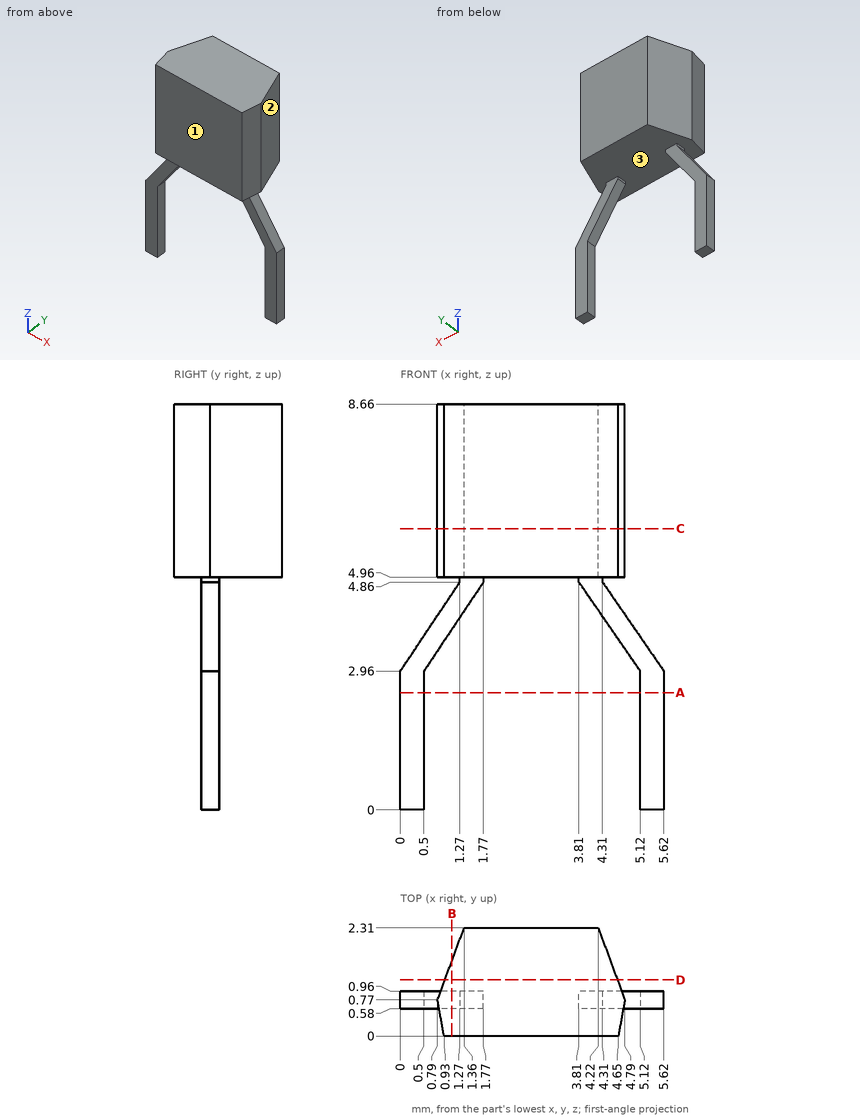
Part print with two shaded views. Sizes in mm from the minimum x, y, z corner. Round coordinates to 2 decimals unless told otherwise and drop trailing zeros. Write each loop counter-clockwise with the first axis right and the second up, starting at its lowest first coordinate (ties: lowest second). Pieces come first, ordered by that corner, then holes. Notation, with made-up numbers: (39.25, 37.5) - (47.25, 37.5) arc R27 cw to (47.25, 69.5) - close; hole circle Ø5 at (-30, 20). An arc over 180 degrees is marked (long way). Answer as CSV lines item,"result".
Q1. Cut at A-A (z = 2.5). Write the cut outline in (x, y), and give its area (3 significant figures).
Report:
outline,"(0, 0.58) - (0.5, 0.58) - (0.5, 0.96) - (0, 0.96) - close; (5.12, 0.58) - (5.62, 0.58) - (5.62, 0.96) - (5.12, 0.96) - close"
area,"0.380 mm^2"
Q2. Pull direction Y, two halves, no side cores. Call the marked faces 1, 2 and 3: +Y half, -Y half, draft (parallel to the pull), parting line (faces both ways), or undercut.
Report:
face 1,"-Y half"
face 2,"+Y half"
face 3,"draft"
Q3. Drop flat-ended pins along their axis: pin 1 (0.9 mm diameter, centred on x = 0.5, z = 2, fed in from +Y); pin 2 (2 mm diameter, centred on x = 3, z = 7, fed in from -Y); pin 3 (1.4 mm diameter, centred on x = 1, z = 2, fed in from -Y). Give the stop position or say it passes through.
Report:
pin 1,"stops at y = 0.96"
pin 2,"stops at y = 0"
pin 3,"stops at y = 0.58"
Q4. Drill centre lines: probe 1 along X at (y, z) = (0.7, 0.5); probe 2 along Z at (x, y) = (1.4, 0.45); probe 3 along Y at (x, z) = (4.45, 4.25). Where is each one in solid material? Low to high. Write a range as [from, to].
Report:
probe 1,"x = [0, 0.5], [5.12, 5.62]"
probe 2,"z = [4.96, 8.66]"
probe 3,"y = [0.58, 0.96]"
Q5. Cut at D-D (y = 1.2). Write the cut outline in (x, z).
Report:
outline,"(0.95, 4.96) - (4.63, 4.96) - (4.63, 8.66) - (0.95, 8.66) - close"
Q6. Cut at C-C (z = 6). Write the cut outline in (x, y), and give its area (3 significant figures).
Report:
outline,"(0.79, 0.77) - (0.93, 0) - (4.65, 0) - (4.79, 0.77) - (4.22, 2.31) - (1.36, 2.31) - close"
area,"8.25 mm^2"
Q7. Cut at B-B (x = 1.1). Write the cut outline in (y, z).
Report:
outline,"(0, 4.96) - (1.61, 4.96) - (1.61, 8.66) - (0, 8.66) - close; (0.58, 3.86) - (0.96, 3.86) - (0.96, 4.61) - (0.58, 4.61) - close"
